Geometry check sheet. Reference: the model listing, model coordinates, mm. Face numbers are marked on the shaded views. A direction names the side the tool comes from. Coordinates: 2 decimals unless noted, no trailing zeros. Loops run counter-clockwise (first coordinate to the right, second up) from the corner with the lowest first, then second, coordinate; pieces in that order, holes last.
from build123d import *

# Parameters (mm, degrees)
BOSS_EXTRUDE2_DEPTH = 5
BOSS_EXTRUDE3_DEPTH = 8
SKETCH4_W           = 4
SKETCH4_H           = 2
CUT_EXTRUDE2_DEPTH  = 2
CUT_EXTRUDE3_DEPTH  = 1
CUT_EXTRUDE4_DEPTH  = 2
BOSS_EXTRUDE4_DEPTH = 1
BOSS_EXTRUDE5_DEPTH = 2


with BuildPart() as part:
    # Sketch1 → Boss-Extrude2 (new body)
    with BuildSketch(Plane.XY):
        with BuildLine():
            Line((4, 2), (4, 6))
            ThreePointArc((4, 6), (1, 9), (-2, 6))
            Line((-2, 6), (-2, 2))
            Line((-2, 2), (-4, 2))
            Line((-4, 2), (-4, -2))
            Line((-4, -2), (4, -2))
            Line((4, -2), (4, 2))
        make_face()
        with BuildLine():
            Line((2, 6), (2, 4))
            ThreePointArc((2, 4), (1, 3), (0, 4))
            Line((0, 4), (0, 6))
            ThreePointArc((0, 6), (1, 7), (2, 6))
        make_face(mode=Mode.SUBTRACT)
    extrude(amount=BOSS_EXTRUDE2_DEPTH)

    # Sketch2 → Boss-Extrude3 (add)
    with BuildSketch(Plane(origin=(4, 0, 0), x_dir=(0, 0, -1), z_dir=(1, 0, 0))):
        with BuildLine():
            Line((-5, -2), (-7, -2))
            Line((-7, -2), (-7, -1))
            ThreePointArc((-7, -1), (-5.545836543, 0.197224362), (-5, 2))
            Line((-5, 2), (-5, -2))
        make_face()
    extrude(amount=-BOSS_EXTRUDE3_DEPTH)

    # Sketch4 → Cut-Extrude2 (cut)
    with BuildSketch(Plane.XZ.offset(2)):
        with Locations((0, 6)):
            Rectangle(SKETCH4_W, SKETCH4_H)
    extrude(amount=-CUT_EXTRUDE2_DEPTH, mode=Mode.SUBTRACT)

    # Sketch5 → Cut-Extrude3 (cut)
    with BuildSketch(Plane.XY.offset(5)):
        with BuildLine():
            Line((4, 6), (2, 6))
            ThreePointArc((2, 6), (1, 7), (0, 6))
            Line((0, 6), (-2, 6))
            ThreePointArc((-2, 6), (1, 9), (4, 6))
        make_face()
    extrude(amount=-CUT_EXTRUDE3_DEPTH, mode=Mode.SUBTRACT)

    # Sketch6 → Cut-Extrude4 (cut)
    with BuildSketch(Plane.XY.offset(5)):
        with BuildLine():
            Line((-2, 4), (-1, 4))
            Line((-1, 4), (-1, 8.236067977))
            ThreePointArc((-1, 8.236067977), (-1.738612788, 7.224744871), (-2, 6))
            Line((-2, 6), (-2, 4))
        make_face()
    extrude(amount=-CUT_EXTRUDE4_DEPTH, mode=Mode.SUBTRACT)

    # Sketch7 → Boss-Extrude4 (add)
    with BuildSketch(Plane(origin=(0, 0, 0), x_dir=(-1, 0, 0), z_dir=(0, 0, -1))):
        Polygon((4, 2), (4, 3), (2, 6), (2, 2), align=None)
    extrude(amount=-BOSS_EXTRUDE4_DEPTH)

    # Sketch8 → Boss-Extrude5 (add)
    with BuildSketch(Plane.ZY.offset(2)):
        Polygon((1, 2), (1, 3), (2, 3), (5, 2), align=None)
    extrude(amount=BOSS_EXTRUDE5_DEPTH)


solid = part.part
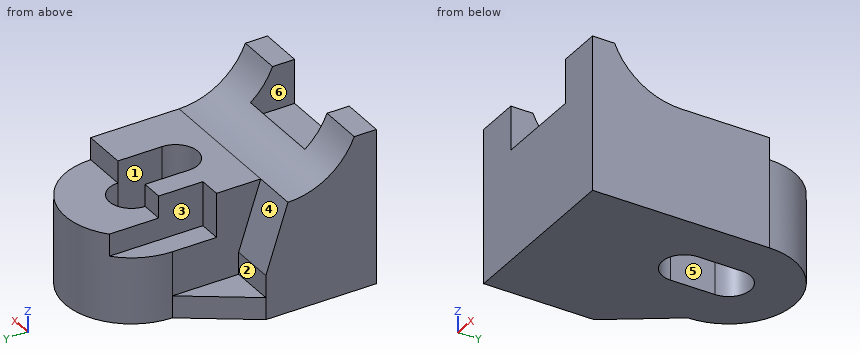
1) Access from +Z, -Z, +X, -X, +Y, -Y to the whole of each face (thin tool, end or side, straight path). Record for the marked faces 4, 5 and 6.
Data:
face 4: +Z, -X, +Y
face 5: +Z, -Z
face 6: +Z, -Y
2) Section check D-D on z = 6.5. Record the cut outline in (x, y).
Data:
outline: (-4, -2) - (-2, -2) - (-2, -0.74) - (-4, -0.74) - close; (2, -2) - (4, -2) - (4, -0.74) - (2, -0.74) - close
3) Section check A-A on y = 5.25. Record the cut outline in (x, z).
Data:
outline: (-2.5, 0) - (0, 0) - (0, 5) - (-1, 5) - (-1, 3) - (-2, 3) - (-2, 1) - (-2.5, 1) - close; (2, 0) - (4, 0) - (4, 5) - (2, 5) - close
4) Mould release check, pull along X, two halves, no side actions. Record for the marked faces 1, 2 and 3: +X half, -X half, draft (parallel to the pull), parting line (faces both ways), or undercut.
Data:
face 1: undercut
face 2: draft
face 3: -X half
5) Section check C-C on x = -3. Record the cut outline in (y, z).
Data:
outline: (-2, 0) - (4.5, 0) - (4.5, 1) - (3, 1) - (3, 2) - (2, 5) arc R3.25 cw to (-1, 7) - (-2, 7) - close
6) Material ranges on probe 1 along Y at (x, z) = (1, 3); probe 2 along Z at (x, y) = (2.5, 8.25); probe 3 along Z at (x, y) = (2.5, 2.5), recorded low to high.
Data:
probe 1: y = -2 to 3, 7 to 9
probe 2: z = 0 to 4
probe 3: z = 0 to 5
7) Section check B-B on x = 1. Record the cut outline in (y, z).
Data:
outline: (-2, 0) - (3, 0) - (3, 5) - (2, 5) arc R3.25 cw to (0, 5.69) - (0, 5) - (-2, 5) - close; (7, 0) - (9, 0) - (9, 4) - (7, 4) - close
8) Depth check by flat-ended pin: pin 1 (4.5 mm diameter, centred on x = 1.5, y = 4, fed in from +Z); pin 2 (0.8 mm diameter, centred on x = -1.5, z = 4, fed in from +Y); pin 3 (1.6 mm diameter, centred on y = 5, z = 2.5, fed in from -X). Enter the tip coordinate at first touch or a pass-through.
Data:
pin 1: stops at z = 5.01
pin 2: stops at y = 4
pin 3: stops at x = -2
